Autodesk Inventor part; units mm, degrees
ref_plane "YZ Plane" through (0, 0, 0) normal (1, 0, 0) x (0, 1, 0)
ref_plane "XZ Plane" through (0, 0, 0) normal (0, 1, 0) x (-1, 0, 0)
ref_plane "XY Plane" through (0, 0, 0) normal (0, 0, 1) x (1, 0, 0)
sketch "Sketch1" plane through (0, 0, 0) normal (0, 0, 1) x (1, 0, 0)
  circle A0 centre (-10.6, 0) radius 8.475
  circle A1 centre (-15.1, 0) radius 2.2
  circle A2 centre (-6.1, 0) radius 2.2
  circle A3 centre (-10.6, 0) radius 8.475
  circle A4 centre (-15.1, 0) radius 2.2
  circle A5 centre (-6.1, 0) radius 2.2
  circle A6 centre (-15.1, 0) radius 1.55
  circle A7 centre (-6.1, 0) radius 1.55
  point P0 (0, 0)
  dimension "d9" = 3.1
  dimension "d10" = 3.1
sketch "Sketch2" plane through (0, 0, 0) normal (0, 1, 0) x (-1, 0, 0)
  line L0 (19.075, 0) -> (2.125, 0)
  line L1 (7.55, 0) -> (13.65, 0)
  arc A0 (18.6, 4) -> (19.075, 0) centre (62.4336, 7.177) ccw
  line L2 (13.65, 0) -> (19.075, 0)
  line L3 (10.6, 0) -> (10.6, 4)
  line L4 (10.6, 0) -> (10.6, 4)
  line L5 (10.6, 4) -> (18.6, 4)
  point P0 (0, 0)
  dimension "d15" = 4
  dimension "d16" = 8
revolve "Revolution1" add sketch "Sketch2" angle 360 about axis through (-10.6, 0, 0) along (0, 0, 1)
extrude "Extrusion3" cut sketch "Sketch1" along normal blind 4 contours A6 | A7
sketch "Sketch5" plane through (-10.6, 0, 4) normal (0, 0, 1) x (1, 0, 0)
  line L0 (1, -3.5) -> (-1, -3.5)
  line L1 (-1, -3.5) -> (-1, 3.5)
  line L2 (-1, 3.5) -> (1, 3.5)
  line L3 (1, 3.5) -> (1, -3.5)
  line L4 (1, -3.5) -> (-1, 3.5) construction
  line L5 (-1, -3.5) -> (1, 3.5) construction
  circle A0 centre (-4.5, 0) radius 1.55
  circle A1 centre (4.5, 0) radius 1.55
  circle A2 centre (-4.5, 0) radius 3
  circle A3 centre (4.5, 0) radius 3
  line L6 (1.25, -1.5) -> (-1.25, -1.5)
  line L7 (-1.25, -1.5) -> (-1.25, 1.5)
  line L8 (-1.25, 1.5) -> (1.25, 1.5)
  line L9 (1.25, 1.5) -> (1.25, -1.5)
  line L10 (1.25, -1.5) -> (-1.25, 1.5) construction
  line L11 (-1.25, -1.5) -> (1.25, 1.5) construction
  point P0 (10.6, 0)
  point P1 (0, 0)
  point P2 (1, -1.5)
  point P3 (1, 1.5)
  point P4 (-1, 1.5)
  point P5 (-1, -1.5)
  dimension "d17" = 2
  dimension "d18" = 7
  dimension "d19" = 6
  dimension "d20" = 6
  dimension "d21" = 2.5
  dimension "d22" = 3
extrude "Extrusion5" cut sketch "Sketch5" against normal blind 4 contours L0 L1 L6 L3 | L6 L1 L8 L3 | L3 L8 L9 L6 | L6 L7 L8 L1 | L8 L1 L2 L3
properties part number "Pot_holder"
Source: CAD feature listing. Evaluate the final solid. Frame: model axes, mm. A direction names the side the tool comes from. Coordinates: 2 decimals unless noted, no trailing zeros. Loops run counter-clockwise (first coordinate to the right, second up) from the corner with the lowest first, then second, coordinate; pieces in that order, holes last. Notation, with made-up numbers: M 88,12.25 L 141,12.25 A5 cw 141,16.25 Z; hole C 28,61.25 d1. An arc over 180 degrees is marked long. Use CSV: the item, a comma, the result in double quotes.
(1) Contact query for flat-ended pins moving along their axis: pin 1 (1 mm diameter, centred on y = -2.5, z = 2.5, fed in from -X); pin 2 (1.6 mm diameter, centred on y = 2, z = 3, fed in from +X); pin 3 (2 mm diameter, centred on x = -10.5, z = 3, fed in from +Y); pin 4 (2.5 mm diameter, centred on x = -15.1, y = 0, fed in from -Z). Output: stop coordinate, or through.
Answers follow:
pin 1,"x = -18.5"
pin 2,"x = -2.58"
pin 3,"y = 8.19"
pin 4,"through"
(2) Cut plane B-B on z = 2.2. Return loops of the section in (x, y).
Answers follow:
outline,"C -10.6,0 d16.34; hole C -15.1,0 d3.1; hole M -11.85,-1.5 L -11.6,-1.5 L -11.6,-3.5 L -9.6,-3.5 L -9.6,-1.5 L -9.35,-1.5 L -9.35,1.5 L -9.6,1.5 L -9.6,3.5 L -11.6,3.5 L -11.6,1.5 L -11.85,1.5 Z; hole C -6.1,0 d3.1"
(3) Reachability of faces 3 (the face through (-11, -3.5, 2)), 4 (the face through (-12, 0, 0)) from +Z, -Z, +X, -X, +Y, -Y: full face, straight path, thin tool, end or side. Return the list, or none.
Answers follow:
face 3,"+Z, -Z"
face 4,"-Z, +X, -X, +Y, -Y"
(4) Draft query along Y for faces 1 (the face through (-11.6, -3, 2)), 2 (the face through (-12, 0, 4)). Return one class per face: pulls with the +Y half, pulls with the -Y half, needs draft (parallel to the pull), parting line crosses it, or undercut.
Answers follow:
face 1,"undercut"
face 2,"needs draft"
(5) Cut plane A-A on y = 0. Return loops of the section in (x, z) (3 decimals), and give its area (3 significant figures).
Answers follow:
outline,"M -19.075,0 L -16.65,0 L -16.65,4 L -18.6,4 A43.947 cw Z; M -13.55,0 L -11.85,0 L -11.85,4 L -13.55,4 Z; M -9.35,0 L -7.65,0 L -7.65,4 L -9.35,4 Z; M -4.55,0 L -2.125,0 A43.947 cw -2.6,4 L -4.55,4 Z"
area,"30.9 mm²"
(6) Line query: line 1 (X direction, y = -0.5, z = 2.5); line 2 (Y direction, x = -15.1, z = 3.05); line 3 (X direction, y = -2.25, z = 3.6). Output: solid intervals per line, ascending. Write a range as [from, to].
Answers follow:
line 1,"[-18.72, -16.57], [-13.63, -11.85], [-9.35, -7.57], [-4.63, -2.48]"
line 2,"[-6.71, -1.55], [1.55, 6.71]"
line 3,"[-18.31, -11.6], [-9.6, -2.89]"
